Job drawing, mm, ordinate dimensions from the low corner. One solid piece. A direction names the side the tool comes from. Give positions to 0.01 mm unless a question says otherwise; leave off trailing zeros. Write each loop counter-clockwise with the first axis right and the second up, starting at its lowest first coordinate (ties: lowest second). Pieces come first, ordered by that corner, then holes. Notation, with made-up numbers: (16, 34.5) - (61, 34.5) arc R23 cw to (61, 67.5) - close; hole circle Ø5 at (23.25, 28). An arc over 180 degrees is marked (long way). Use a Markdown table: item, result. Add a question column.
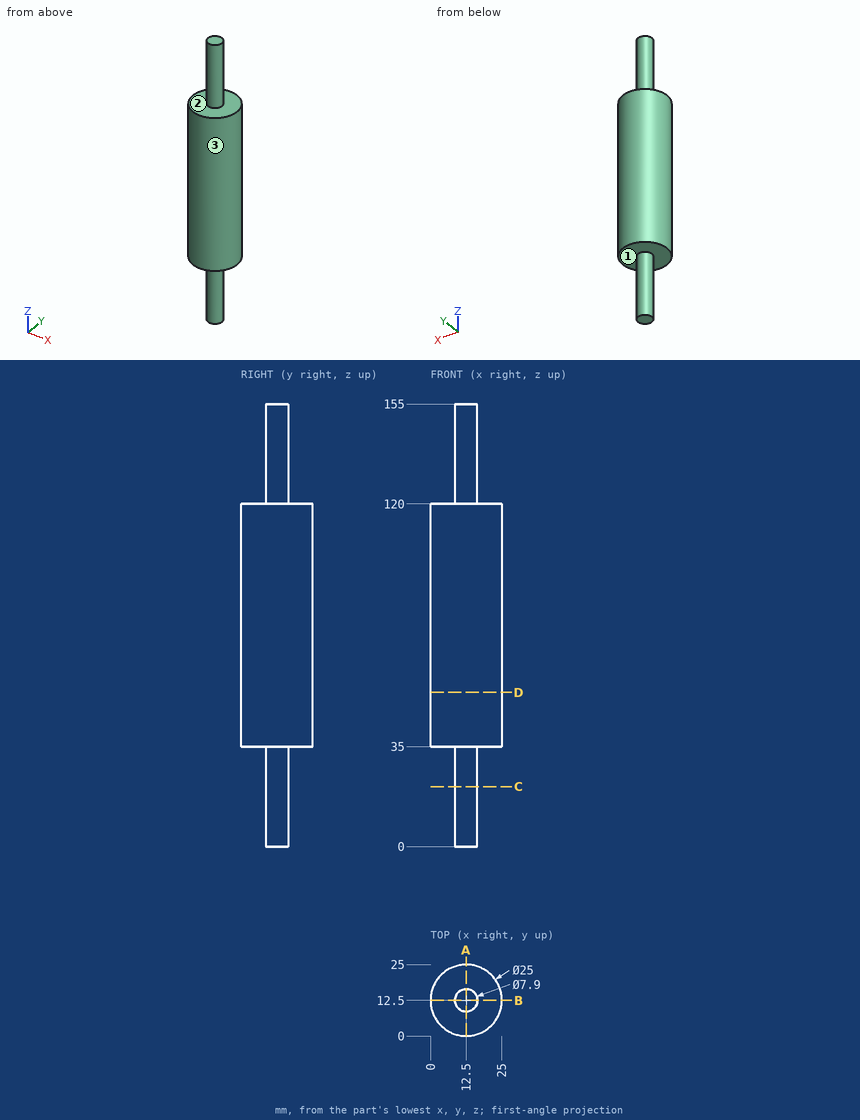
(1) Band-saw the part on C-C (z = 21). Write the cut outline in (x, y).
(2) Which spindle directions (+Z, -Z, +X, -X, +Y, -Y) get a long thin tool onto all of the face, cutting with end or side? Do the marked faces 1, 2 and 3. Say none if no direction does.
(3) Flat gauge pins, fed straight in: pin 1 (3 mm diameter, centred on y = 7, z = 101.5, fed in from -X); pin 2 (12 mm diameter, centred on y = 6.5, z = 64, fed in from +X); pin 3 (8 mm diameter, centred on x = 13, z = 20.5, fed in from +Y); pin 4 (5 mm diameter, centred on y = 14.5, z = 123, fed in from +X). Where does each tip first touch, or does it go through?
(4) Band-saw the part on D-D (z = 54). Write the cut outline in (x, y), then the cut area to 3 significant figures.
(5) Probe probe 1 along Y at (x, z) = (12.5, 61.5); probe 2 along Z at (x, y) = (22.5, 19); probe 3 along Y at (x, z) = (21.75, 46). List the from-to ranges inside material, lowest first. Write a range as [from, to].
(6) Band-saw the part on A-A (x = 12.5). Write the cut outline in (y, z).
Model answer:
| question | item | result |
|---|---|---|
| 1 | outline | circle Ø7.9 at (12.5, 12.5) |
| 2 | face 1 | -Z |
| 2 | face 2 | +Z |
| 2 | face 3 | +Z, -Z |
| 3 | pin 1 | stops at x = 0.66 |
| 3 | pin 2 | stops at x = 25 |
| 3 | pin 3 | stops at y = 16.45 |
| 3 | pin 4 | stops at x = 16.45 |
| 4 | outline | circle Ø25 at (12.5, 12.5) |
| 4 | area | 491 mm^2 |
| 5 | probe 1 | y = [0, 25] |
| 5 | probe 2 | z = [35, 120] |
| 5 | probe 3 | y = [4.09, 20.91] |
| 6 | outline | (0, 35) - (8.55, 35) - (8.55, 0) - (16.45, 0) - (16.45, 35) - (25, 35) - (25, 120) - (16.45, 120) - (16.45, 155) - (8.55, 155) - (8.55, 120) - (0, 120) - close |
